```python
from build123d import *

# Parameters (mm, degrees)
SKETCH1_R           = 1.999999943
BOSS_EXTRUDE1_DEPTH = 6
SKETCH1_3_R         = 1.999999943
BOSS_EXTRUDE2_DEPTH = 8.54


with BuildPart() as part:
    # Sketch1 → Boss-Extrude1 (new body)
    with BuildSketch(Plane.XY):
        with BuildLine():
            Line((-19.553972123, -40.529522255), (-21.543248991, -49.954902644))
            Line((-21.543248991, -49.954902644), (-20.41822196, -50.425046499))
            ThreePointArc((-20.41822196, -50.425046499), (-10.404121129, -53.396800588), (-0.006635132, -54.399707743))
            ThreePointArc((-0.006635132, -54.399707743), (10.39066306, -53.396824107), (20.404594428, -50.42516399))
            Line((20.404594428, -50.42516399), (21.529621459, -49.955020135))
            Line((21.529621459, -49.955020135), (19.54391785, -40.534371527))
            ThreePointArc((19.54391785, -40.534371527), (-0.005581304, -44.999999654), (-19.553972123, -40.529522255))
        make_face()
        with Locations((-16.665975394, -46.501988883)):
            Circle(SKETCH1_R, mode=Mode.SUBTRACT)
        with Locations((16.665975394, -46.501988883)):
            Circle(SKETCH1_R, mode=Mode.SUBTRACT)
    extrude(amount=BOSS_EXTRUDE1_DEPTH)

    # Sketch1_3 → Boss-Extrude2 (add)
    with BuildSketch(Plane.XY):
        with Locations((-16.665975394, -46.501988883)):
            Circle(SKETCH1_3_R)
        with Locations((16.665975394, -46.501988883)):
            Circle(SKETCH1_3_R)
        with BuildLine():
            Line((-20.41822196, -50.425046499), (-21.543248991, -49.954902644))
            Line((-21.543248991, -49.954902644), (-21.669150988, -50.551438115))
            ThreePointArc((-21.669150988, -50.551438115), (-0.006892589, -54.999999568), (21.656480116, -50.556867674))
            Line((21.656480116, -50.556867674), (21.529621459, -49.955020135))
            Line((21.529621459, -49.955020135), (20.404594428, -50.42516399))
            ThreePointArc((20.404594428, -50.42516399), (10.39066306, -53.396824107), (-0.006635132, -54.399707743))
            ThreePointArc((-0.006635132, -54.399707743), (-10.404121129, -53.396800588), (-20.41822196, -50.425046499))
        make_face()
    extrude(amount=BOSS_EXTRUDE2_DEPTH)


solid = part.part
```
Design review of the part built by this model. Coordinates are the model's own, in mm. A direction names the side the tool comes from. Coordinates: 2 decimals unless noted, no trailing zeros. Order: outer loops, then holes, each group sorted by start corner. A loop starts at its lowest first (then second) coordinate and runs counter-clockwise, first axis right, second up. Notation, with made-up numbers: (36, 52.5) - (77, 52.5) arc R22 ccw to (77, 70.5) - close; hole circle Ø4 at (-26, -10). An arc over 180 degrees is marked (long way). One line per question, with ' | ' between items.
Q1. For faces 1 (the flat face through (20.97, -50.19, 7.25)), 2 (the cylindrical face through (16.41, -44.52, 7.25)), 3 (the flat face through (-17, -46, 8.54)), list the 3-axis set-ups (+Z, -Z, +X, -X, +Y, -Y) from which the entire face can be reached by the end or side of a thin tool; tool diameter is ignored.
Answer key:
face 1: +Z, +Y | face 2: +Z | face 3: +Z, +X, -X, +Y, -Y
Q2. Consider section C-C, the plane x = 18. Give the boundary of the cut face in (y, z), then the cut area to 3 significant figures.
Answer key:
outline: (-51.97, 0) - (-41.24, 0) - (-41.24, 6) - (-45.01, 6) - (-45.01, 8.54) - (-47.99, 8.54) - (-47.99, 6) - (-51.33, 6) - (-51.33, 8.54) - (-51.97, 8.54) - close | area: 73.6 mm2
Q3. Clearance check with flat-ended pins moving along their axes: pin 1 Ø6 at (x, y) = (-12.5, -50.5) entering from +Z; pin 2 Ø4 at (y, z) = (-43, 1.5) entering from +X; pin 3 Ø3 at (y, z) = (-50.5, 2.5) entering from +X; pin 4 Ø2 at (x, z) = (-6.5, 3.5) entering from -Y. State where each tip first meets the part, or that it passes through.
Answer key:
pin 1: stops at z = 8.54 | pin 2: stops at x = 20.49 | pin 3: stops at x = 21.66 | pin 4: stops at y = -54.72
Q4. Consider section B-B, the plane z = 6.5. Give the boundary of the cut face in (x, y), then the cut area to 3 significant figures.
Answer key:
outline: (-21.67, -50.55) arc R55 ccw to (21.66, -50.56) - (21.53, -49.96) - (20.4, -50.43) arc R54.4 cw to (-20.42, -50.43) - (-21.54, -49.95) - close; circle Ø4 at (-16.67, -46.5); circle Ø4 at (16.67, -46.5) | area: 51.8 mm2
Q5. Consider section D-D, the plane y = -52.25. Give the boundary of the cut face in (x, z).
Answer key:
outline: (-17.17, 0) - (17.17, 0) - (17.17, 8.54) - (15.13, 8.54) - (15.13, 6) - (-15.15, 6) - (-15.15, 8.54) - (-17.17, 8.54) - close
Q6. The part is to be moulded in two halves that separate along X. For faces 4 (the cylindrical face through (0, -45, 3)), 5 (the cylindrical face through (0, -55, 4)), 6 (the flat face through (0, -48, 0)), say which applies: +X half, -X half, draft (parallel to the pull), parting line (faces both ways), or undercut.
Answer key:
face 4: undercut | face 5: parting line | face 6: draft
Q7. To check wall thickness, follow line 1 along Z through (x, y) = (-18, -41.75); line 2 along X through (y, z) = (-47.75, 7); line 3 along Y through (x, z) = (-5, 6.5). State the ranges of each line that lie inside material, in increasing order.
Answer key:
line 1: z = 0 to 6 | line 2: x = -18.23 to -15.1, 15.1 to 18.23 | line 3: y = -54.77 to -54.17
